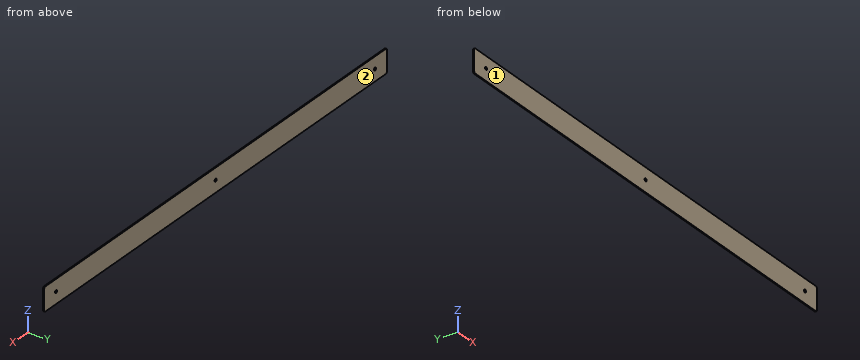
```python
from build123d import *

# Parameters (mm, degrees)
SKETCH1_W           = 636.566333418
SKETCH1_H           = 31.75
BOSS_EXTRUDE1_DEPTH = 1.524
SKETCH2_R           = 1.905
CUT_EXTRUDE1_DEPTH  = 2.524
FILLET1_R           = 2.54


with BuildPart() as part:
    # Sketch1 → Boss-Extrude1 (new body)
    with BuildSketch(Plane(origin=(0, 0, 0), x_dir=(1, 0, 0), z_dir=(0, 1, 0))):
        Rectangle(SKETCH1_W, SKETCH1_H)
    extrude(amount=BOSS_EXTRUDE1_DEPTH)

    # Sketch2 → Cut-Extrude1 (cut, through all)
    with BuildSketch(Plane(origin=(0, 1.524, 0), x_dir=(1, 0, 0), z_dir=(0, 1, 0))):
        with Locations((-296.164, 0)):
            Circle(SKETCH2_R)
        with Locations((296.164, 0)):
            Circle(SKETCH2_R)
        Circle(SKETCH2_R)
    extrude(amount=-CUT_EXTRUDE1_DEPTH, mode=Mode.SUBTRACT)

    # Fillet1
    fillet1_edges = [part.edges().sort_by_distance(p)[0] for p in [
        (318.283166709, 0.762, 15.875),
        (-318.283166709, 0.762, 15.875),
        (-318.283166709, 0.762, -15.875),
        (318.283166709, 0.762, -15.875),
    ]]
    fillet(fillet1_edges, radius=FILLET1_R)


solid = part.part
```
Source: CAD feature listing. Evaluate the final solid. Frame: model axes, mm. Face numbers are marked on the shaded views. Round coordinates to 2 decimals unless told otherwise and drop trailing zeros. Use CSV: the item, a comma, the result in double quotes.
Q1. Ray query, line 1 along X through (y, z) = (0.45, 0) (3 decimals); line 2 along Z through (x, y) = (0, 0.5) (3 decimals); line 3 along X through (y, z) = (0.35, -14). Return the intervals inside material, ascending.
Reported:
line 1,"-318.283 to -298.069, -294.259 to -1.905, 1.905 to 294.259, 298.069 to 318.283"
line 2,"-15.875 to -1.905, 1.905 to 15.875"
line 3,"-318.19 to 318.19"
Q2. Pin query (flat end, axial travel): pin 1 Ø4.5 at (x, z) = (296.164, 0) entering from -Y; pin 2 Ø3 at (x, z) = (0, 0) entering from -Y. Return the tip coordinate at first contact, or that it passes through.
Reported:
pin 1,"y = 0"
pin 2,"through"
Q3. Mould query, pull axis Y, two halves, no side actions, for the marked faces 1 and 2. Classes: pulls with the +Y half, pulls with the -Y half, needs draft (parallel to the pull), parting line crosses it, or undercut.
Reported:
face 1,"pulls with the -Y half"
face 2,"pulls with the +Y half"
